from build123d import *

# Parameters (mm, degrees)
F0_R     = 9
F1_DEPTH = 140
F2_DEPTH = 100
F4_DEPTH = 10.751
F5_COUNT = 3
F0_R_2   = 2.25
F6_DEPTH = 4
F7_START = 46
F7_DEPTH = 4
F8_START = 62
F0_R_3   = 7.5
F8_DEPTH = 3


# Not quite as in the source:
# - a feature names something its author has since deleted; it is built from what else it names


with BuildPart() as f1:
    # F0 (on Top) → F1 (new body)
    with BuildSketch(Plane.XY):
        with BuildLine():
            ThreePointArc((-3, -9.5393920142), (-2.2464281062, -9.744411771), (-1.4791551643, -9.89))
            ThreePointArc((-1.4791551643, -9.89), (0, -10), (1.4791551643, -9.89))
            ThreePointArc((1.4791551643, -9.89), (2.2464281062, -9.744411771), (3, -9.5393920142))
            ThreePointArc((3, -9.5393920142), (8.0622577483, -5.9160797831), (10, 0))
            ThreePointArc((10, 0), (7.3314391493, 6.8007352544), (0.75, 9.9718353376))
            ThreePointArc((0.75, 9.9718353376), (0, 10), (-0.75, 9.9718353376))
            ThreePointArc((-0.75, 9.9718353376), (-9.9341644436, 1.1455901566), (-3, -9.5393920142))
        make_face()
        Circle(F0_R, mode=Mode.SUBTRACT)
    extrude(amount=F1_DEPTH)

    # F0 (on Top) → F2 (join)
    with BuildSketch(Plane.XY):
        with BuildLine():
            Line((-0.75, 34.9718353376), (-0.75, 9.9718353376))
            ThreePointArc((-0.75, 9.9718353376), (0, 10), (0.75, 9.9718353376))
            Line((0.75, 9.9718353376), (0.75, 34.9718353376))
            Line((0.75, 34.9718353376), (-0.75, 34.9718353376))
        make_face()
    extrude(amount=F2_DEPTH)

    # F3 (on face) → F4 (cut, through all)
    with BuildSketch(Plane.YZ.offset(0.75)):
        with BuildLine():
            Line((34.9718353376, 100), (9.9718353376, 100))
            Line((9.9718353376, 100), (9.9718353376, 94.1647440576))
            add(Edge.make_bspline(
                [(9.9718353376, 94.1647440576), (10.1832449594, 91.2204140215), (12.0836351221, 77.2918027042), (20.9708053433, 61.8272021249), (33.801245613, 48.6414831262), (34.7842815391, 38.599508776), (34.9718353376, 32.702038365)],
                knots=[0.0899218527, 0.0899218527, 0.0899218527, 0.0899218527, 0.2371904705, 0.3995520788, 0.5544857931, 0.7015059428, 0.7015059428, 0.7015059428, 0.7015059428], degree=3))
            Line((34.9718353376, 32.702038365), (34.9718353376, 100))
        make_face()
    extrude(amount=-F4_DEPTH, mode=Mode.SUBTRACT)


with BuildPart() as f5_1:
    # F5: instance of F1
    add(f1.part.rotate(Axis((0, 0, 0), (0, 0, 1)), 1 * 360 / F5_COUNT))


with BuildPart() as f5_2:
    # F5: instance of F1
    add(f1.part.rotate(Axis((0, 0, 0), (0, 0, 1)), 2 * 360 / F5_COUNT))


with BuildPart() as f1_1:
    add(f1.part)

    add(f5_1.part)  # F6 merges F5_1

    add(f5_2.part)  # F6 merges F5_2
    # F0 (on Top) → F6 (join)
    with BuildSketch(Plane.XY):
        with BuildLine():
            ThreePointArc((1.4791551643, -9.89), (0, -10), (-1.4791551643, -9.89))
            ThreePointArc((-1.4791551643, -9.89), (-2.592051841, -10.9896135416), (-3, -12.5))
            ThreePointArc((-3, -12.5), (0, -15.5), (3, -12.5))
            ThreePointArc((3, -12.5), (2.592051841, -10.9896135416), (1.4791551643, -9.89))
        make_face()
        with Locations((0, -12.5)):
            Circle(F0_R_2, mode=Mode.SUBTRACT)
        with BuildLine():
            ThreePointArc((-3, -12.5), (-2.592051841, -10.9896135416), (-1.4791551643, -9.89))
            ThreePointArc((-1.4791551643, -9.89), (-2.2464281062, -9.744411771), (-3, -9.5393920142))
            Line((-3, -9.5393920142), (-3, -12.5))
        make_face()
        with BuildLine():
            ThreePointArc((3, -9.5393920142), (2.2464281062, -9.744411771), (1.4791551643, -9.89))
            ThreePointArc((1.4791551643, -9.89), (2.592051841, -10.9896135416), (3, -12.5))
            Line((3, -12.5), (3, -9.5393920142))
        make_face()
    extrude(amount=F6_DEPTH)

    # F0 (on Top) → F7 (join)
    with BuildSketch(Plane.XY.offset(F7_START)):
        with BuildLine():
            ThreePointArc((1.4791551643, -9.89), (0, -10), (-1.4791551643, -9.89))
            ThreePointArc((-1.4791551643, -9.89), (-2.592051841, -10.9896135416), (-3, -12.5))
            ThreePointArc((-3, -12.5), (0, -15.5), (3, -12.5))
            ThreePointArc((3, -12.5), (2.592051841, -10.9896135416), (1.4791551643, -9.89))
        make_face()
        with Locations((0, -12.5)):
            Circle(F0_R_2, mode=Mode.SUBTRACT)
        with BuildLine():
            ThreePointArc((-3, -12.5), (-2.592051841, -10.9896135416), (-1.4791551643, -9.89))
            ThreePointArc((-1.4791551643, -9.89), (-2.2464281062, -9.744411771), (-3, -9.5393920142))
            Line((-3, -9.5393920142), (-3, -12.5))
        make_face()
        with BuildLine():
            ThreePointArc((3, -9.5393920142), (2.2464281062, -9.744411771), (1.4791551643, -9.89))
            ThreePointArc((1.4791551643, -9.89), (2.592051841, -10.9896135416), (3, -12.5))
            Line((3, -12.5), (3, -9.5393920142))
        make_face()
    extrude(amount=F7_DEPTH)

    # F0 (on Top) → F8 (join)
    with BuildSketch(Plane.XY.offset(F8_START)):
        Circle(F0_R)
        Circle(F0_R_3, mode=Mode.SUBTRACT)
    extrude(amount=F8_DEPTH)


solid = f1_1.part
Could you check a few things on this model? Use its own coordinates, in mm. A direction names the side the tool comes from. Round coordinates to 2 decimals unless told otherwise and drop trailing zeros. Write each loop counter-clockwise with the first axis right and the second up, starting at its lowest first coordinate (ties: lowest second). Pieces come first, ordered by that corner, then holes. Notation, with made-up numbers: (25, -23) - (54, -23) arc R19 cw to (54, -4) - close; hole circle Ø10 at (-8, -19.75). An arc over 180 degrees is marked (long way). Use a Markdown table: item, result.
Q1. For pin 1 (12 mm diameter, centred on y = -5, z = 60.5, fed in from +X); pin 2 (1.5 mm diameter, centred on y = -6, z = 59, fed in from +X); pin 3 (20 mm diameter, centred on y = 27.5, z = 36, fed in from -X), each with a flat end and sliding along its axis, tell me the tip position at first contact or that it passes through.
Output values:
| item | result |
|---|---|
| pin 1 | x = 20.53 |
| pin 2 | x = 13.19 |
| pin 3 | x = -0.75 |
Q2. Thinking about a two-plate mould opening in Y: for faces 6 (the flat face through (-2, 7.4, 65)), 7 (the cylindrical face through (-1.172, 8.923, 30.566)), 8 (the flat face through (18.935, -11.798, 35.96)), 9 (the flat face through (2, -11, 50)), which applies, released by +Y, released by -Y, zero draft, split by the parting line, or undercut?
Output values:
| item | result |
|---|---|
| face 6 | undercut |
| face 7 | undercut |
| face 8 | released by -Y |
| face 9 | zero draft |
Q3. Please list where these lines run through material, in increasing order: L1, parallel to Y at x = 0, z = 2.5; L2, parallel to X at y = -12, z = 47; L3, parallel to Y at x = 0, z = 31.
Output values:
| item | result |
|---|---|
| L1 | -15.5 to -14.75, -10.25 to -9, 9 to 34.97 |
| L2 | -22.28 to -19.28, -3 to -2.19, 2.19 to 3, 19.28 to 22.28 |
| L3 | -10 to -9, 9 to 34.97 |
Q4. I want a section at A-A (z = 17.5). List the corners of the cut face in (x, y) for me.
Output values:
| item | result |
|---|---|
| outline | (-30.66, -16.84) - (-29.91, -18.14) - (-8.26, -5.64) arc R10 ccw to (8.26, -5.64) - (29.91, -18.14) - (30.66, -16.84) - (9.01, -4.34) arc R10 ccw to (0.75, 9.97) - (0.75, 34.97) - (-0.75, 34.97) - (-0.75, 9.97) arc R10 ccw to (-9.01, -4.34) - close; hole circle Ø18 at (0, 0) |
Q5. For faces 1 (the cylindrical face through (-1.172, 8.923, 101.975)), 2 (the flat face through (-3, -11, 48)), 3 (the flat face through (-9.2, 0.7, 0)), 4 (the flat face through (-0.75, 23, 36)), 5 (the flat face through (0.75, 22, 36)), which set-ups out of +Z, -Z, +X, -X, +Y, -Y let a thin tool reach every point of the face, with its end or its side?
Output values:
| item | result |
|---|---|
| face 1 | +Z |
| face 2 | +Z, -Z, -Y |
| face 3 | -Z, +X, -X, +Y, -Y |
| face 4 | +Z, -Z, -X, +Y |
| face 5 | +Z, -Z, +X, +Y |
